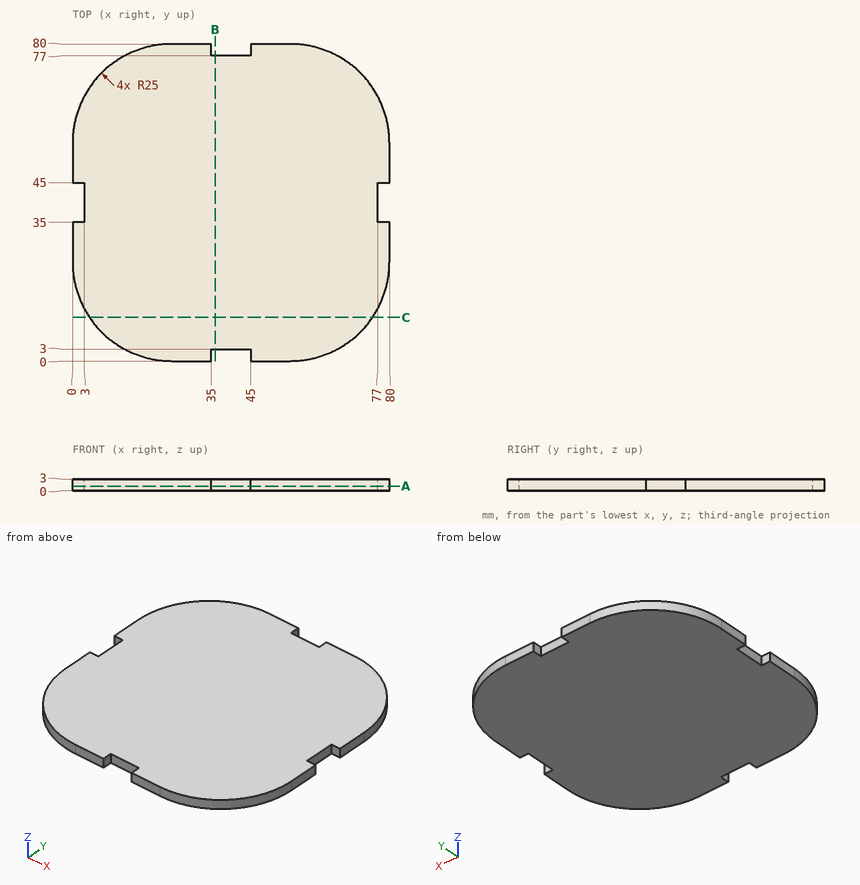
Source: three-view drawing plus pictorial views. Frame: mm from the lowest corner of the part. Round coordinates to 2 decimals unless told otherwise and drop trailing zeros. Loops run counter-clockwise (first coordinate to the right, second up) from the corner with the lowest first, then second, coordinate; pieces in that order, holes last.
Q1. Section A-A on z = 1.2. Return loops of the section in (x, y), plus the area to 3 significant figures.
Q2. Section C-C on y = 11. Return loops of the section in (x, z), plus the area to 3 significant figures.
Q3. Material intervals for L1, parallel to X at y = 38.5, z = 2.5; L2, parallel to X at y = 57, z = 0.45, sorted ascending.
Q4. Section B-B on x = 36. Return loops of the section in (y, z), plus the area to 3 significant figures.
Q5. Pin query (flat end, axial travel): P1, Ø1.5, axis at x = 1.5, z = 2, coming from the +Y side; P2, Ø0.9, axis at y = 78.5, z = 2, coming from the +X side; P3, Ø1.5, axis at y = 40.5, z = 1, coming from the -X side. Return the tip coordinate at first contact, or that it passes through.
Evaluation:
1. outline: (0, 25) arc R25 ccw to (25, 0) - (35, 0) - (35, 3) - (45, 3) - (45, 0) - (55, 0) arc R25 ccw to (80, 25) - (80, 35) - (77, 35) - (77, 45) - (80, 45) - (80, 55) arc R25 ccw to (55, 80) - (45, 80) - (45, 77) - (35, 77) - (35, 80) - (25, 80) arc R25 ccw to (0, 55) - (0, 45) - (3, 45) - (3, 35) - (0, 35) - close
1. area: 5,740 mm2
2. outline: (4.29, 0) - (75.71, 0) - (75.71, 3) - (4.29, 3) - close
2. area: 214 mm2
3. L1: x = 3 to 77
3. L2: x = 0.08 to 79.92
4. outline: (3, 0) - (77, 0) - (77, 3) - (3, 3) - close
4. area: 222 mm2
5. P1: stops at y = 65.37
5. P2: stops at x = 64.68
5. P3: stops at x = 3
